Part model, mm, in its own coordinate system. Face numbers are marked on the shaded views. Coordinates: 2 decimals unless noted, no trailing zeros. Order: outer loops, then holes, each group sorted by start corner. A loop starts at its lowest first (then second) coordinate and runs counter-clockwise, first axis right, second up.
Autodesk Inventor part; units mm, degrees
ref_plane "Work Plane1" through (8.7, 0, 2) normal (0, 0, -1) x (-1, 0, 0)
ref_plane "YZ Plane" through (0, 0, 0) normal (1, 0, 0) x (0, 1, 0)
ref_plane "XZ Plane" through (0, 0, 0) normal (0, 1, 0) x (-1, 0, 0)
sketch "Sketch1" plane through (0, 0, 0) normal (0, 0, 1) x (1, 0, 0)
  circle A0 centre (8.7, 0) radius 3.375
  circle A1 centre (8.7, 0) radius 6.5
  circle A2 centre (8.7, 0) radius 4.75
  point P0 (0, 0)
  dimension "d0" = 13
  dimension "d1" = 9.5
extrude "Extrusion1" add sketch "Sketch1" along normal blind 3.5 and the other way blind 0.5 contours A1
ref_plane "Work Plane1" through (8.7, 0, 2) normal (0, 0, -1) x (-1, 0, 0)
sketch "Sketch2" plane through (8.7, 0, 2) normal (0, 0, -1) x (-1, 0, 0)
  circle A0 centre (0, 0) radius 6.5
  circle A1 centre (0, 0) radius 4.75
  circle A2 centre (0, 0) radius 5.5
  circle A3 centre (-5.5, 0) radius 2.25
  line L0 (-7.75, 0) -> (-3.25, 0)
  point P0 (8.7, 0)
  dimension "d5" = 11
  dimension "d6" = 4.5
revolve "Revolution1" cut sketch "Sketch2" angle 360 about axis through (16.45, 0, 2) along (-1, 0, 0) picked at (-6.8857, -0.4037) picked at (-5.7999, -1.7269) picked at (-5.2327, -0.251) picked at (-4.2505, -0.3733) contours A3 L0 A0 | A0 L0 A2 A3 | A2 L0 A1 A3 | A1 L0 A3
pattern_circular "Circular Pattern1" count 5 over 360 about axis through (8.7, 0, 3.5) along (0, 0, -1) of "Revolution1"
properties part number "Hex Bearing Spacer"
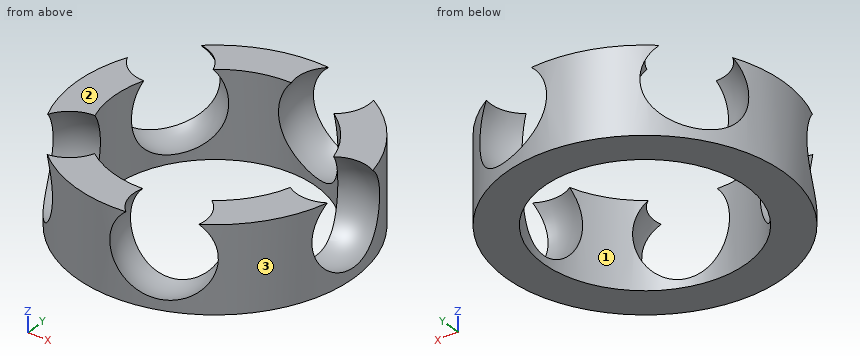
Q1. Cut at D-D on z = 3.1. Write the cut outline in (x, y), and give its area (3 significant figures).
Results list:
outline: (2.58, -2.2) arc R1.96 cw to (4.12, -1.27) arc R4.75 cw to (4.12, 1.27) arc R1.96 cw to (2.58, 2.2) arc R6.5 ccw to start; (4.72, -5.14) arc R6.5 ccw to (8.9, -6.5) arc R1.96 cw to (8.5, -4.75) arc R4.75 cw to (6.07, -3.96) arc R1.96 cw to start; (4.72, 5.14) arc R1.96 cw to (6.07, 3.96) arc R4.75 cw to (8.5, 4.75) arc R1.96 cw to (8.9, 6.5) arc R6.5 ccw to start; (11.65, -3.72) arc R1.96 cw to (12.36, -5.37) arc R6.5 ccw to (14.94, -1.82) arc R1.96 cw to (13.15, -1.66) arc R4.75 cw to start; (11.65, 3.72) arc R4.75 cw to (13.15, 1.66) arc R1.96 cw to (14.94, 1.82) arc R6.5 ccw to (12.36, 5.37) arc R1.96 cw to start
area: 28.3 mm2
Q2. Cut at C-C on y = -4.5. Write the cut outline in (x, z), and give its area (3 significant figures).
Results list:
outline: (4.01, -0.5) - (7.18, -0.5) - (7.18, 3.5) - (5.35, 3.5) arc R1.86 cw to (4.01, 0.16) - close; (10.22, -0.5) - (13.39, -0.5) - (13.39, 3.5) - (11.91, 3.5) arc R2.13 cw to (10.22, -0.12) - close
area: 12.3 mm2
Q3. Cut at A-A on z = 0.4. Write the cut outline in (x, y).
Results list:
outline: (2.77, -2.67) arc R1.58 cw to (4.25, -1.65) arc R4.75 cw to (4.25, 1.65) arc R1.58 cw to (2.77, 2.67) arc R6.5 ccw to start; (4.33, -4.81) arc R6.5 ccw to (9.41, -6.46) arc R1.58 cw to (8.89, -4.75) arc R4.75 cw to (5.75, -3.73) arc R1.58 cw to start; (4.33, 4.81) arc R1.58 cw to (5.75, 3.73) arc R4.75 cw to (8.89, 4.75) arc R1.58 cw to (9.41, 6.46) arc R6.5 ccw to start; (11.33, -3.95) arc R1.58 cw to (11.93, -5.64) arc R6.5 ccw to (15.06, -1.33) arc R1.58 cw to (13.27, -1.28) arc R4.75 cw to start; (11.33, 3.95) arc R4.75 cw to (13.27, 1.28) arc R1.58 cw to (15.06, 1.33) arc R6.5 ccw to (11.93, 5.64) arc R1.58 cw to start
Q4. Mould opens along X. For the marked faces 1, 2 and 3 say: pulls with the +X half, pulls with the -X half, needs draft (parallel to the pull), parting line crosses it, or undercut.
Results list:
face 1: undercut
face 2: needs draft
face 3: parting line crosses it
Q5. Wall check: line 1 along Z through (x, y) = (12.5, 4); line 2 along X through (y, z) = (0, 2.5); line 3 along Y through (x, z) = (6.25, 1.3). Give the ranges that are in metal, low to high.
Results list:
line 1: z = -0.5 to 3.5
line 2: x = 2.2 to 3.95
line 3: y = -6.02 to -4.07, 4.07 to 6.02
Q6. Cut at B-B on x = 7.5. Write the cut outline in (y, z).
Results list:
outline: (-6.39, -0.5) - (-4.6, -0.5) - (-4.6, 3.5) - (-6.39, 3.5) - close; (4.6, -0.5) - (6.39, -0.5) - (6.39, 3.5) - (4.6, 3.5) - close
Q7. Pin check, flat tips, straight feed: pin 1 Ø1.8 at (x, y) = (13, -2.5) entering from +Z; pin 2 Ø1 at (y, z) = (-1, 0.5) entering from +X; pin 3 Ø1.5 at (x, z) = (13.5, 3) entering from -Y. Stop position of each tip, or through.
Results list:
pin 1: stops at z = 3.5
pin 2: stops at x = 15.16
pin 3: stops at y = -5.08
